```python
from build123d import *

# Parameters (mm, degrees)
SKETCH3_W           = 33.274
SKETCH3_H           = 33.274
SKETCH3_R           = 9.525
SKETCH3_R_2         = 1.651
BOSS_EXTRUDE1_DEPTH = 3.175
CUT_EXTRUDE1_DEPTH  = 24.741528236
SKETCH5_R           = 10.7315
SKETCH5_R_2         = 9.525
BOSS_EXTRUDE2_DEPTH = 2.032
FILLET1_R           = 3.81


with BuildPart() as part:
    # Sketch3 → Boss-Extrude1 (new body)
    with BuildSketch(Plane.XY):
        Rectangle(SKETCH3_W, SKETCH3_H)
        Circle(SKETCH3_R, mode=Mode.SUBTRACT)
        with Locations((-13.47089, 13.47089)):
            Circle(SKETCH3_R_2, mode=Mode.SUBTRACT)
        with Locations((-13.47089, -13.47089)):
            Circle(SKETCH3_R_2, mode=Mode.SUBTRACT)
        with Locations((13.47089, 13.47089)):
            Circle(SKETCH3_R_2, mode=Mode.SUBTRACT)
        with Locations((13.47089, -13.47089)):
            Circle(SKETCH3_R_2, mode=Mode.SUBTRACT)
    extrude(amount=BOSS_EXTRUDE1_DEPTH)

    # Sketch4 → Cut-Extrude1 (cut, through all)
    with BuildSketch(Plane.XY.offset(3.175)):
        with BuildLine():
            Line((-8.980761939, 16.637), (-8.980761939, 13.47089))
            Line((-8.980761939, 13.47089), (-5.938925744, 10.429053805))
            ThreePointArc((-5.938925744, 10.429053805), (0, 12.0015), (5.938925744, 10.429053805))
            Line((5.938925744, 10.429053805), (8.980761939, 13.47089))
            Line((8.980761939, 13.47089), (8.980761939, 16.637))
            Line((8.980761939, 16.637), (-8.980761939, 16.637))
        make_face()
        with BuildLine():
            Line((-16.637, 8.980761939), (-13.47089, 8.980761939))
            Line((-13.47089, 8.980761939), (-10.429053805, 5.938925744))
            ThreePointArc((-10.429053805, 5.938925744), (-12.0015, 0), (-10.429053805, -5.938925744))
            Line((-10.429053805, -5.938925744), (-13.47089, -8.980761939))
            Line((-13.47089, -8.980761939), (-16.637, -8.980761939))
            Line((-16.637, -8.980761939), (-16.637, 8.980761939))
        make_face()
        with BuildLine():
            Line((-8.980761939, -16.637), (-8.980761939, -13.47089))
            Line((-8.980761939, -13.47089), (-5.938925744, -10.429053805))
            ThreePointArc((-5.938925744, -10.429053805), (0, -12.0015), (5.938925744, -10.429053805))
            Line((5.938925744, -10.429053805), (8.980761939, -13.47089))
            Line((8.980761939, -13.47089), (8.980761939, -16.637))
            Line((8.980761939, -16.637), (-8.980761939, -16.637))
        make_face()
        with BuildLine():
            Line((16.637, -8.980761939), (13.47089, -8.980761939))
            Line((13.47089, -8.980761939), (10.429053805, -5.938925744))
            ThreePointArc((10.429053805, -5.938925744), (12.0015, 0), (10.429053805, 5.938925744))
            Line((10.429053805, 5.938925744), (13.47089, 8.980761939))
            Line((13.47089, 8.980761939), (16.637, 8.980761939))
            Line((16.637, 8.980761939), (16.637, -8.980761939))
        make_face()
    extrude(amount=-CUT_EXTRUDE1_DEPTH, mode=Mode.SUBTRACT)

    # Sketch5 → Boss-Extrude2 (add)
    with BuildSketch(Plane.XY.offset(3.175)):
        with Locations(Location((0, 0, 0), (0, 0, 180))):
            Circle(SKETCH5_R)
        Circle(SKETCH5_R_2, mode=Mode.SUBTRACT)
    extrude(amount=BOSS_EXTRUDE2_DEPTH)

    # Fillet1
    fillet1_edges = [part.edges().sort_by_distance(p)[0] for p in [
        (8.980761939, 13.47089, 1.5875),
        (5.938925744, 10.429053805, 1.5875),
        (-5.938925744, 10.429053805, 1.5875),
        (-8.980761939, 13.47089, 1.5875),
        (-13.47089, 8.980761939, 1.5875),
        (-10.429053805, 5.938925744, 1.5875),
        (-10.429053805, -5.938925744, 1.5875),
        (-13.47089, -8.980761939, 1.5875),
        (-8.980761939, -13.47089, 1.5875),
        (-5.938925744, -10.429053805, 1.5875),
        (5.938925744, -10.429053805, 1.5875),
        (8.980761939, -13.47089, 1.5875),
        (13.47089, -8.980761939, 1.5875),
        (10.429053805, -5.938925744, 1.5875),
        (10.429053805, 5.938925744, 1.5875),
        (13.47089, 8.980761939, 1.5875),
    ]]
    fillet(fillet1_edges, radius=FILLET1_R)


solid = part.part
```
Can you work these out from the model? Positions are in its coordinate system, mm. A direction names the side the tool comes from. Coordinates: 2 decimals unless noted, no trailing zeros. Write each loop counter-clockwise with the first axis right and the second up, starting at its lowest first coordinate (ties: lowest second). Pieces come first, ordered by that corner, then holes. Notation, with made-up numbers: (40, -0.75) - (75, -0.75) arc R25 ccw to (75, 37.25) - close; hole circle Ø1 at (32, -5.5). An arc over 180 degrees is marked (long way). Return JSON: item names as keys, results as strings.
Q1. I'm going to push flat-ended pins straight in: pin 1 Ø2 at (y, z) = (5, 4.5) entering from -X; pin 2 Ø5.5 at (x, y) = (-13.47, 13.47) entering from +Z (3 decimals). Where does each tip first touch, or does it pass through?
Computed values:
{"pin 1": "stops at x = -9.96", "pin 2": "stops at z = 3.175"}
Q2. Thinking about a two-plate mould opening in X: for faces 4 (the cylindrical face through (-11.266, 5.984, 1.565)), 5 (the flat face through (-16, 8.981, 2)), 6 (the cylindrical face through (0, -12, 2)), which applies, +X half, -X half, draft (parallel to the pull), parting line (faces both ways), or undercut?
Computed values:
{"face 4": "-X half", "face 5": "draft", "face 6": "undercut"}
Q3. Please list where these lines run through material, in increasing order: L1, parallel to Y at x = 14, z = 2.55; L2, parallel to X at y = 15.5, z = 1.2; L3, parallel to X at y = 7.5, z = 4.3. Write a range as from..to.
Computed values:
{"L1": "y = -16.64..-15.03, -11.91..-8.83, 8.83..11.91, 15.03..16.64", "L2": "x = -16.64..-8.98, 8.98..16.64", "L3": "x = -7.68..-5.87, 5.87..7.68"}
Q4. If we section it at A-A (x = 0): Please give me the cut outline in (y, z) (1 decimal).
Computed values:
{"outline": "(-12, 0) - (-9.5, 0) - (-9.5, 5.2) - (-10.7, 5.2) - (-10.7, 3.2) - (-12, 3.2) - close; (9.5, 0) - (12, 0) - (12, 3.2) - (10.7, 3.2) - (10.7, 5.2) - (9.5, 5.2) - close"}
Q5. On a 3-axis mill with a long thin cutter (end or side, diameter ignored), from which of +Z, -Z, +X, -X, +Y, -Y can I reach the whole of each face in a straight line? I mean faces 1 (the cylindrical face through (-8.7, -13.61, 1.57)), 2 (the flat face through (16, -8.981, 2)), 3 (the flat face through (8.981, 16, 2)). Say none if no direction works.
Computed values:
{"face 1": "+Z, -Z, -Y", "face 2": "+Z, -Z, +X", "face 3": "+Z, -Z, +Y"}
Q6. If we section it at D-D (x = -10): Please give me the cut outline in (y, z) (3 decimals).
Computed values:
{"outline": "(-16.637, 0) - (16.637, 0) - (16.637, 3.175) - (3.894, 3.175) - (3.894, 5.207) - (-3.894, 5.207) - (-3.894, 3.175) - (-16.637, 3.175) - close"}
